```python
from build123d import *

# Parameters (mm, degrees)
SKETCH1_W                 = 246
SKETCH1_H                 = 106
BOSS_EXTRUDE1_DEPTH       = 12
SKETCH3_R                 = 2
CUT_EXTRUDE1_DEPTH        = 50.25
LPATTERN1_COUNT           = 2
LPATTERN1_PITCH           = 31
LPATTERN1_COPY_1_SKETCH_R = 2
LPATTERN1_COPY_1_DEPTH    = 50.25
LPATTERN2_COUNT           = 2
LPATTERN2_PITCH           = 161
MIRROR2_COPY_1_SKETCH_R   = 2
MIRROR2_COPY_1_DEPTH      = 50.25
MIRROR2_COPY_2_SKETCH_R   = 2
MIRROR2_COPY_2_DEPTH      = 50.25


with BuildPart() as part:
    # Sketch1 → Boss-Extrude1 (new body)
    with BuildSketch(Plane(origin=(0, 0, 0), x_dir=(1, 0, 0), z_dir=(0, 1, 0))):
        Polygon((-135, 65), (135, 65), (135, -65), (-135, -65), (-169.840376894, -65), (-169.840376894, 65), align=None)
        with Locations((-21.947414212, 0)):
            Rectangle(SKETCH1_W, SKETCH1_H, mode=Mode.SUBTRACT)
    extrude(amount=BOSS_EXTRUDE1_DEPTH)

    # Sketch3 → Cut-Extrude1 (cut)
    with BuildSketch(Plane(origin=(0, 12, 0), x_dir=(1, 0, 0), z_dir=(0, 1, 0))):
        with Locations(Location((-65.5, -59, 0), (0, 0, 270))):
            Circle(SKETCH3_R)
    cut_extrude1 = extrude(amount=-CUT_EXTRUDE1_DEPTH, mode=Mode.SUBTRACT)

    # Mirror1: Cut-Extrude1 across plane
    add(cut_extrude1.mirror(Plane.XY), mode=Mode.SUBTRACT)

    # LPattern1: Cut-Extrude1 ×2
    with Locations(*[(i * LPATTERN1_PITCH, 0, 0) for i in range(1, LPATTERN1_COUNT)]):
        add(cut_extrude1, mode=Mode.SUBTRACT)

    # LPattern1 copy 1 sketch → LPattern1 copy 1 (cut)
    with BuildSketch(Plane(origin=(31, 12, 0), x_dir=(1, 0, 0), z_dir=(0, 1, 0))):
        with Locations((-65.5, 59)):
            Circle(LPATTERN1_COPY_1_SKETCH_R)
    extrude(amount=-LPATTERN1_COPY_1_DEPTH, mode=Mode.SUBTRACT)

    # LPattern2: Cut-Extrude1 ×2
    with Locations(*[(i * LPATTERN2_PITCH, 0, 0) for i in range(1, LPATTERN2_COUNT)]):
        add(cut_extrude1, mode=Mode.SUBTRACT)

    # Mirror2 copy 1 sketch → Mirror2 copy 1 (cut)
    with BuildSketch(Plane(origin=(161, 12, 0), x_dir=(1, 0, 0), z_dir=(0, 1, 0))):
        with Locations((-65.5, 59)):
            Circle(MIRROR2_COPY_1_SKETCH_R)
    extrude(amount=-MIRROR2_COPY_1_DEPTH, mode=Mode.SUBTRACT)

    # Mirror2 copy 2 sketch → Mirror2 copy 2 (cut)
    with BuildSketch(Plane(origin=(0, 12, 0), x_dir=(1, 0, 0), z_dir=(0, 1, 0))):
        with Locations((-65.5, 59)):
            Circle(MIRROR2_COPY_2_SKETCH_R)
    extrude(amount=-MIRROR2_COPY_2_DEPTH, mode=Mode.SUBTRACT)


solid = part.part
```
Read the model definition and answer for the solid it produces. Units are mm, in the model's axes. A direction names the side the tool comes from. Give positions to 0.01 mm unless a question says otherwise; leave off trailing zeros. Loops run counter-clockwise (first coordinate to the right, second up) from the corner with the lowest first, then second, coordinate; pieces in that order, holes last.
Item 1: For faces 1 (the flat face through (-24, 6, -53)), 2 (the flat face through (-15, 12, 57)), determine the directions among +Z, -Z, +X, -X, +Y, -Y from which every point of the face is accessible in a straight line to the end or side of a thin tool.
Item 2: The part is cut by section B-B (x = -135). Write down the section's boundary in (y, z).
Item 3: This flat-tipped pin is pushed along its axis until it touches: pin 1 Ø2.5 at (x, z) = (-65.5, -59) entering from -Y. Where does it stop, or does it pass through?
Item 4: Find the intervals of material crossed by line 1 along X through (y, z) = (6, 59); line 2 along Z through (x, y) = (-57, 8.75); line 3 along X through (y, z) = (11.25, -30), in increasing order.
Item 5: The mould has two halves that part along Z. Classify faces 3 (the flat face through (-20, 6, 65)), 4 (the flat face through (-24, 6, 53)), 5 (the flat face through (-144.947, 6, 1)), 6 (the flat face through (-15, 6, -65)): released by +Z, released by -Z, zero draft, split by the parting line, or undercut.
Item 6: The part is cut by section C-C (y = 5). Write down the section's boundary in (x, z), and give its area (3 significant figures).
Item 7: The part is cut by section A-A (z = 6.5). Write down the section's boundary in (x, y).
Taken from the geometry:
1. face 1: +Y, -Y
1. face 2: +Z, -Z, +X, -X, +Y
2. outline: (0, -65) - (12, -65) - (12, -53) - (0, -53) - close; (0, 53) - (12, 53) - (12, 65) - (0, 65) - close
3. pin 1: passes through
4. line 1: x = -169.84 to -67.5, -63.5 to -36.5, -32.5 to 93.5, 97.5 to 135
4. line 2: z = -65 to -53, 53 to 65
4. line 3: x = -169.84 to -144.95, 101.05 to 135
5. face 3: released by +Z
5. face 4: undercut
5. face 5: undercut
5. face 6: released by -Z
6. outline: (-169.84, -65) - (135, -65) - (135, 65) - (-169.84, 65) - close; hole (-144.95, -53) - (101.05, -53) - (101.05, 53) - (-144.95, 53) - close; hole circle Ø4 at (-65.5, -59); hole circle Ø4 at (-65.5, 59); hole circle Ø4 at (-34.5, -59); hole circle Ø4 at (-34.5, 59); hole circle Ø4 at (95.5, -59); hole circle Ø4 at (95.5, 59)
6. area: 13,500 mm2
7. outline: (-169.84, 0) - (-144.95, 0) - (-144.95, 12) - (-169.84, 12) - close; (101.05, 0) - (135, 0) - (135, 12) - (101.05, 12) - close
